CAD build for the part. Positions are in the model's coordinates, mm. Round coordinates to 2 decimals unless told otherwise and drop trailing zeros. Write each loop counter-clockwise with the first axis right and the second up, starting at its lowest first coordinate (ties: lowest second). Pieces come first, ordered by that corner, then holes. Notation, with made-up numbers: (38.5, 49.5) - (88.5, 49.5) arc R19 ccw to (88.5, 66.5) - close; hole circle Ø7 at (80, 68.5). An arc over 180 degrees is marked (long way). Put each result on its own line as item: value. Start each with the question number.
Item 1: Cut at A-A (y = -4.5). Give the cut face in (x, z), and give its area (3 significant figures).
Item 2: Cut at B-B (z = 25). Give the cut face in (x, y), and give its area (3 significant figures).
Item 3: Drill centre lines: line 1 (X direction, y = 62.5, z = 18); line 2 (X direction, y = 35.5, z = 29); line 3 (X direction, y = -35.5, z = 17.5). Where is each one in solid material? Low to high. Write a range as from..to.
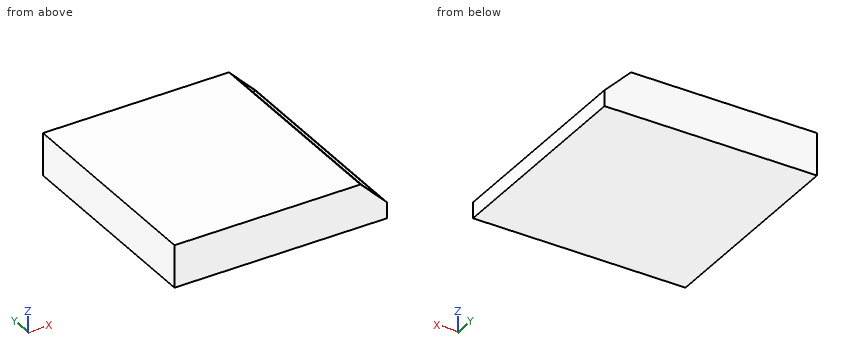
```python
from build123d import *

# Parameters (mm, degrees)
PAD_DEPTH    = 100
SKETCH001_W  = 25
SKETCH001_H  = 190
POCKET_DEPTH = 2


with BuildPart() as part:
    # Sketch → Pad (new body, symmetric)
    with BuildSketch(Plane.XZ):
        Polygon((-100, 40), (-100, 0), (100, 0), (100, 15), (75, 40), align=None)
    extrude(amount=PAD_DEPTH, both=True)

    # Sketch001 (on DatumPlane) → Pocket (cut)
    with BuildSketch(Plane(origin=(100, -100, 15), x_dir=(-0.707107, 0, 0.707107), z_dir=(0.707107, 0, 0.707107))):
        with Locations((17.5, -100.241764)):
            Rectangle(SKETCH001_W, SKETCH001_H)
    extrude(amount=-POCKET_DEPTH, mode=Mode.SUBTRACT)


solid = part.part
```
Output values:
1. outline: (-100, 0) - (100, 0) - (100, 15) - (96.46, 18.54) - (95.05, 17.12) - (77.37, 34.8) - (78.79, 36.21) - (75, 40) - (-100, 40) - close
1. area: 7,640 mm2
2. outline: (-100, -100) - (90, -100) - (90, -94.76) - (87.17, -94.76) - (87.17, 95.24) - (90, 95.24) - (90, 100) - (-100, 100) - close
2. area: 37,500 mm2
3. line 1: -100..94.17, 95.93..97
3. line 2: -100..83.17
3. line 3: -100..94.67, 95.43..97.5
